Read the model definition and answer for the solid it produces. Units are mm, in the model's axes. A direction names the side the tool comes from. Coordinates: 2 decimals unless noted, no trailing zeros. Loops run counter-clockwise (first coordinate to the right, second up) from the corner with the lowest first, then second, coordinate; pieces in that order, holes last. Notation, with made-up numbers: M 39,-25.75 L 78,-25.75 A22 cw 78,0.25 Z; hole C 59,86.25 d11. An arc over 180 degrees is marked long. One line per item, written item: value. Start each with the question number.
1. The part is cut by section C-C (x = 0). Write down the section's boundary in (y, z).
2. The part is cut by section A-A (y = -0.75). Write down the section's boundary in (x, z), then the cut area to 3 significant figures.
3. Consider probe 1 along Z at (x, y) = (0, -5.5); probe 2 along Z at (x, y) = (0, -3); probe 3 along X at (y, z) = (-2, -1). Determine where each line is inside the solid, lowest interval first.
4. Determine the mould class of faces 1 (the face through (27.55, -3.45, -27.57)), 2 (the face through (-0.81, -3.55, -17.16)), 3 (the face through (0, -7, 0)) for opening direction X: +X half, -X half, draft (parallel to the pull), parting line (faces both ways), or undercut.
5. Flat-ended cylindrical pins translate along their axes: pin 1 (3 mm diameter, centred on x = -18, z = 9, fed in from +Y); pin 2 (7 mm diameter, centred on x = 0, z = -13.5, fed in from -Y). Find the tip coordinate at first contact, or state that the pin passes through.
6. The part is cut by section D-D (x = 19). Write down the section's boundary in (y, z).
7. The part is cut by section B-B (z = -13.5). Write down the section's boundary in (x, y).
8. For faces 4 (the face through (0, -4, 0)), 5 (the face through (0, -3, 28)), determine the directions among +Z, -Z, +X, -X, +Y, -Y from which every point of the face is accessible in a straight line to the end or side of a thin tool.
```python
from build123d import *

# Parameters (mm, degrees)
F1_DEPTH = 7
F2_R     = 3.75
F3_DEPTH = 7
F4_T     = -3


with BuildPart() as f1:
    # F0 (on Front) → F1 (new body)
    with BuildSketch(Plane.XZ):
        with BuildLine():
            ThreePointArc((28, 26.5), (27.56066, 27.56066), (26.5, 28))
            Line((26.5, 28), (-26.5, 28))
            ThreePointArc((-26.5, 28), (-27.56066, 27.56066), (-28, 26.5))
            Line((-28, 26.5), (-28, -26.5))
            ThreePointArc((-28, -26.5), (-27.56066, -27.56066), (-26.5, -28))
            Line((-26.5, -28), (26.5, -28))
            ThreePointArc((26.5, -28), (27.56066, -27.56066), (28, -26.5))
            Line((28, -26.5), (28, 26.5))
        make_face()
    extrude(amount=F1_DEPTH)

    # F2 (on face) → F3 (cut)
    with BuildSketch(Plane.XZ.offset(7)):
        with Locations((0, -13.5)):
            Circle(F2_R)
    extrude(amount=-F3_DEPTH, mode=Mode.SUBTRACT)

    # F4
    f4_openings = [f1.faces().sort_by_distance(p)[0] for p in [
        (0, 0, 0.19302),
    ]]
    offset(amount=F4_T, openings=f4_openings)


solid = f1.part
```
Answer block:
1. outline: M -7,-28 L 0,-28 L 0,-25 L -4,-25 L -4,-20.25 L 0,-20.25 L 0,-17.25 L -7,-17.25 Z; M -7,-9.75 L 0,-9.75 L 0,-6.75 L -4,-6.75 L -4,25 L 0,25 L 0,28 L -7,28 Z
2. outline: M -28,-26.5 A1.5 ccw -26.5,-28 L 26.5,-28 A1.5 ccw 28,-26.5 L 28,26.5 A1.5 ccw 26.5,28 L -26.5,28 A1.5 ccw -28,26.5 Z; C 0,-13.5 d13.5; hole M -25,-25 L 25,-25 L 25,25 L -25,25 Z; hole C 0,-13.5 d7.5
2. area: 733 mm2
3. probe 1: z = -28 to -17.25, -9.75 to 28
3. probe 2: z = -28 to -25, -20.25 to -17.25, -9.75 to -6.75, 25 to 28
3. probe 3: x = -28 to -25, 25 to 28
4. face 1: +X half
4. face 2: undercut
4. face 3: draft
5. pin 1: stops at y = -4
5. pin 2: passes through
6. outline: M -7,-28 L 0,-28 L 0,-25 L -4,-25 L -4,25 L 0,25 L 0,28 L -7,28 Z
7. outline: M -28,-7 L -3.75,-7 L -3.75,0 L -6.75,0 L -6.75,-4 L -25,-4 L -25,0 L -28,0 Z; M 3.75,-7 L 28,-7 L 28,0 L 25,0 L 25,-4 L 6.75,-4 L 6.75,0 L 3.75,0 Z
8. face 4: +Y
8. face 5: +Z, +X, -X, +Y, -Y
